```python
from build123d import *

# Parameters (mm, degrees)
EXTRUDE_1_DEPTH     = 27
SKETCH_2_W          = 55
SKETCH_2_H          = 14
CUT_EXTRUDE_1_DEPTH = 27
SKETCH_3_W          = 52
SKETCH_3_H          = 16
CUT_EXTRUDE_2_DEPTH = 90
CUT_EXTRUDE_START   = -19
SKETCH_4_R          = 12.5
CUT_EXTRUDE_3_DEPTH = 19
CUT_EXTRUDE_4_DEPTH = 20
SKETCH_6_R          = 1.05
CUT_EXTRUDE_5_DEPTH = 65.158008074


with BuildPart() as part:
    # 草图1 → 凸台-拉伸1 (new body)
    with BuildSketch(Plane(origin=(0, 0, 0), x_dir=(1, 0, 0), z_dir=(0, 1, 0))):
        with BuildLine():
            Line((-32, -46.5), (32, -46.5))
            ThreePointArc((32, -46.5), (34.121320344, -45.621320344), (35, -43.5))
            Line((35, -43.5), (35, 43.5))
            ThreePointArc((35, 43.5), (34.121320344, 45.621320344), (32, 46.5))
            Line((32, 46.5), (-32, 46.5))
            ThreePointArc((-32, 46.5), (-34.121320344, 45.621320344), (-35, 43.5))
            Line((-35, 43.5), (-35, -43.5))
            ThreePointArc((-35, -43.5), (-34.121320344, -45.621320344), (-32, -46.5))
        make_face()
    extrude(amount=EXTRUDE_1_DEPTH)

    # 草图2 → 切除-拉伸1 (cut)
    with BuildSketch(Plane.ZY.offset(35)):
        with Locations((-9, 10)):
            Rectangle(SKETCH_2_W, SKETCH_2_H)
    extrude(amount=-CUT_EXTRUDE_1_DEPTH, mode=Mode.SUBTRACT)

    # 草图3 → 切除-拉伸2 (cut)
    with BuildSketch(Plane.XY.offset(46.5)):
        with Locations((0, 16)):
            Rectangle(SKETCH_3_W, SKETCH_3_H)
    extrude(amount=-CUT_EXTRUDE_2_DEPTH, mode=Mode.SUBTRACT)

    # 草图4 → 切除-拉伸3 (cut)
    with BuildSketch(Plane(origin=(0, 27, 0), x_dir=(1, 0, 0), z_dir=(0, 1, 0)).offset(CUT_EXTRUDE_START)):
        with Locations(Location((3, 13.5, 0), (0, 0, 270))):
            Circle(SKETCH_4_R)
        with BuildLine():
            Line((26, 40.5), (22, 40.5))
            ThreePointArc((22, 40.5), (19.878679656, 39.621320344), (19, 37.5))
            Line((19, 37.5), (19, -16.5))
            Line((19, -16.5), (14, -16.5))
            Line((14, -16.5), (14, -21.5))
            Line((14, -21.5), (19, -21.5))
            Line((19, -21.5), (26, -21.5))
            ThreePointArc((26, -21.5), (28.121320344, -20.621320344), (29, -18.5))
            Line((29, -18.5), (29, 37.5))
            ThreePointArc((29, 37.5), (28.121320344, 39.621320344), (26, 40.5))
        make_face()
    extrude(amount=CUT_EXTRUDE_3_DEPTH, mode=Mode.SUBTRACT)

    # 草图5 → 切除-拉伸4 (cut)
    with BuildSketch(Plane(origin=(0, 0, 18.5), x_dir=(-1, 0, 0), z_dir=(0, 0, -1))):
        Polygon((26, 17), (30, 17), (30, 3), (8, 3), (8, 8), (26, 8), align=None)
    extrude(amount=-CUT_EXTRUDE_4_DEPTH, mode=Mode.SUBTRACT)

    # 草图6 → 切除-拉伸5 (cut, through all)
    with BuildSketch(Plane(origin=(0, 27, 0), x_dir=(1, 0, 0), z_dir=(0, 1, 0))):
        with Locations(Location((-32, 43, 0), (0, 0, 270))):
            Circle(SKETCH_6_R)
        with Locations(Location((-32, -43, 0), (0, 0, 270))):
            Circle(SKETCH_6_R)
        with Locations(Location((32, -43, 0), (0, 0, 270))):
            Circle(SKETCH_6_R)
        with Locations(Location((32, 43, 0), (0, 0, 270))):
            Circle(SKETCH_6_R)
    extrude(amount=-CUT_EXTRUDE_5_DEPTH, mode=Mode.SUBTRACT)


solid = part.part
```
Build history of the part. All positions in model axes, mm. A direction names the side the tool comes from. Round coordinates to 2 decimals unless told otherwise and drop trailing zeros. Write each loop counter-clockwise with the first axis right and the second up, starting at its lowest first coordinate (ties: lowest second). Pieces come first, ordered by that corner, then holes.
1) Pin check, flat tips, straight feed: pin 1 (4 mm diameter, centred on x = -5.5, z = -14, fed in from +Y); pin 2 (8 mm diameter, centred on x = 0, y = 19.5, fed in from +Z). Stop position of each tip, or through.
2) Band-saw the part on B-B, the plane x = 10.5. List the corners of the cut face in (y, z).
3) Drill centre lines: probe 1 along X at (y, z) = (11.75, -43); probe 2 along X at (y, z) = (25.4, -13.5); probe 3 along Z at (x, y) = (3, 25.65). Where is each one in solid material? Low to high.
4) 3-axis set-ups, long thin cutter, end or side, ignore diameter. For faces 1 (the cylindrical face through (-31.95, 13.69, -44.05)), 2 (the flat face through (-33, 10, 18.5)), 3 (the flat face through (24, 25, -40.5)), 4 (the flat face through (26, 16, 34)): which of +Z, -Z, +X, -X, +Y, -Y reach the whole face in a straight line?
5) Band-saw the part on C-C, the plane z = -23.5. List the corners of the cut face in (x, y).
6) Band-saw the part on A-A, the plane y = 9.5. List the corners of the cut face in (x, z), and give its area (3 significant figures).
7) Mould opens along Y. For faces 5 (the flat face through (-31, 17, 0)), 6 (the flat face through (0, 27, -1)), 7 (the cylindrical face through (11.45, 25.48, -22.71)) say: +Y half, -Y half, draft (parallel to the pull), parting line (faces both ways), or undercut.
8) Band-saw the part on D-D, the plane x = -21.5. List the corners of the cut face in (y, z), and give its area (3 significant figures).
Ans:
1. pin 1: stops at y = 8
1. pin 2: stops at z = -43.5
2. outline: (0, -46.5) - (27, -46.5) - (27, -23.5) - (24, -23.5) - (24, -43.5) - (8, -43.5) - (8, 46.5) - (0, 46.5) - close; (24, -3.5) - (27, -3.5) - (27, 46.5) - (24, 46.5) - close
3. probe 1: x = -35 to -33.05, -30.95 to -26, 26 to 30.95, 33.05 to 35
3. probe 2: x = -35 to -9.5, 15.5 to 19, 29 to 35
3. probe 3: z = -46.5 to -26, -1 to 46.5
4. face 1: +Y, -Y
4. face 2: -X
4. face 3: +Y
4. face 4: +Z
5. outline: (-35, 0) - (35, 0) - (35, 27) - (29, 27) - (29, 8) - (-8, 8) - (-8, 3) - (-35, 3) - close; (-35, 17) - (-26, 17) - (-26, 24) - (-4.5, 24) - (-4.5, 27) - (-35, 27) - close; (10.5, 24) - (19, 24) - (19, 27) - (10.5, 27) - close
6. outline: (-35, -43.5) arc R3 ccw to (-32, -46.5) - (32, -46.5) arc R3 ccw to (35, -43.5) - (35, 43.5) arc R3 ccw to (32, 46.5) - (26, 46.5) - (26, 21.5) arc R3 cw to (29, 18.5) - (29, -37.5) arc R3 cw to (26, -40.5) - (26, -43.5) - (-26, -43.5) - (-26, -36.5) - (-35, -36.5) - close; (-35, 18.5) - (-30, 18.5) - (-30, 38.5) - (-26, 38.5) - (-26, 46.5) - (-32, 46.5) arc R3 ccw to (-35, 43.5) - close; hole circle Ø2.1 at (-32, -43); hole circle Ø2.1 at (-32, 43); hole circle Ø2.1 at (32, -43); hole circle Ø2.1 at (32, 43)
6. area: 1,050 mm2
7. face 5: undercut
7. face 6: +Y half
7. face 7: draft
8. outline: (0, -46.5) - (27, -46.5) - (27, 46.5) - (24, 46.5) - (24, -43.5) - (8, -43.5) - (8, -36.5) - (3, -36.5) - (3, 38.5) - (8, 38.5) - (8, 46.5) - (0, 46.5) - close
8. area: 696 mm2
